Study the drawing (mm; zero at the part's minimum x, y, z) and answer. A direction names the side the tool comes from. Give positions to 0.01 mm unless a question says otherwise; leave off trailing zeros. Write each loop counter-clockwise with the first axis right and the second up, starting at its lowest first coordinate (ties: lowest second). Pieces come first, ordered by that corner, then holes. Notation, with made-up numbers: (-32.5, -30) - (-28.5, -30) arc R9 cw to (-28.5, -18) - close; hole circle Ø10 at (15.5, -38). An arc over 180 degrees is marked (long way). Answer in a Markdown table with one row per item. Add a question column.
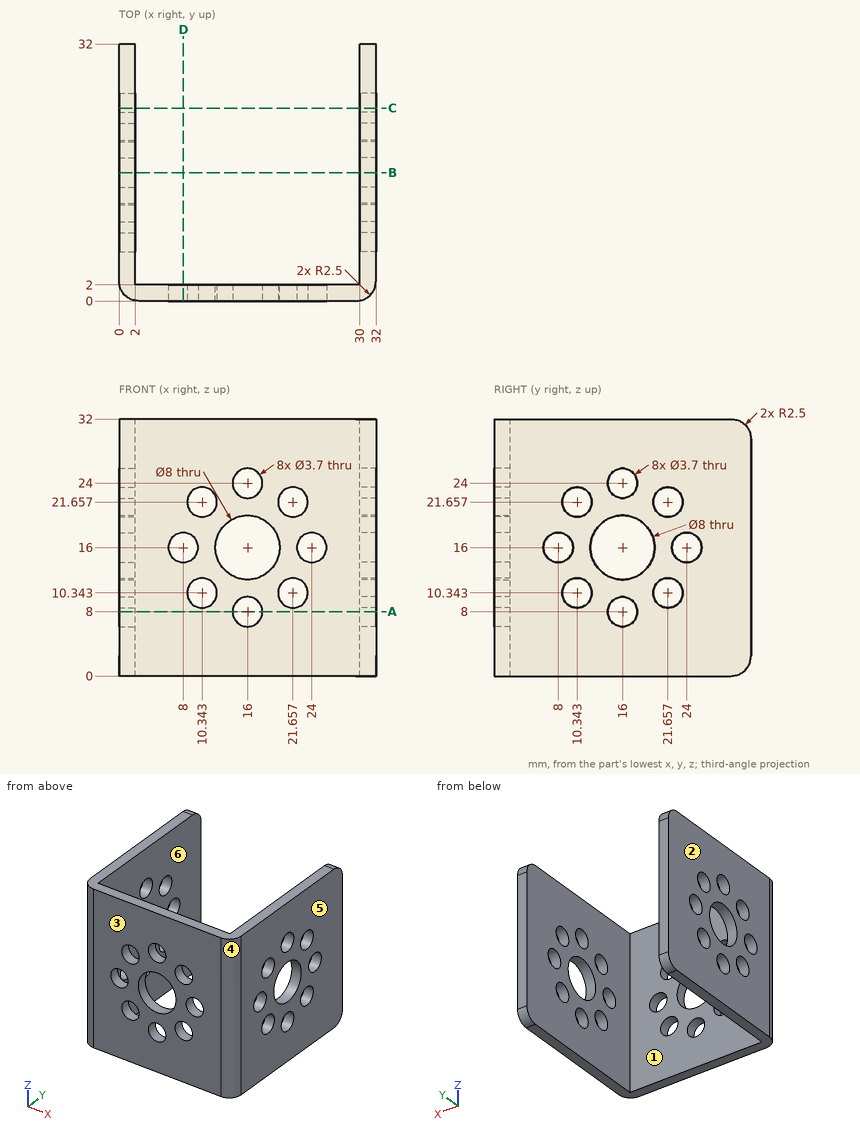
1. Section A-A (z = 8) is taken. Give the vertices of the cut face in (x, y), and give its area (3 significant figures).
2. Section D-D (x = 8) is taken. Give the vertices of the cut face in (y, z), and give its area (3 significant figures).
3. Section B-B (y = 16) is taken. State how many separate pieces and enclosed holes the cut face has, and give its area (3 significant figures).
4. The mould has two halves that part along X. Classify the marked faces 1, 2, 3 and 4: +X half, -X half, draft (parallel to the pull), parting line (faces both ways), or undercut.
5. Given pin 1 Ø3 at (y, z) = (24, 16) entering from -X; pin 2 Ø1 at (x, z) = (17.5, 4) entering from +Y, each flat-ended and moving along its own axis, determine where each tip first touches the part or whether it passes through.
6. Straight lines are drawn through the part: L1, parallel to Z at x = 16, y = 1.05; L2, parallel to X at y = 2.5, z = 2.5; L3, parallel to Y at x = 31, z = 16. For each, find the intervals that lie inside material, in ascending order. Write a range as [from, to].
7. Section C-C (y = 24) is taken. Give the vertices of the cut face in (x, z), and give its area (3 significant figures).
8. A tool of negligible diameter and unlimited length cuts with its end or side. For the marked faces 5 and 6, from which of +Z, -Z, +X, -X, +Y, -Y can it reach the whole face along a straight path? Write none if from no direction.
Geometry check:
| question | item | result |
|---|---|---|
| 1 | outline | (0, 2.5) arc R2.5 ccw to (2.5, 0) - (14.15, 0) - (14.15, 2) - (2, 2) - (2, 14.15) - (0, 14.15) - close; (0, 17.85) - (2, 17.85) - (2, 32) - (0, 32) - close; (17.85, 0) - (29.5, 0) arc R2.5 ccw to (32, 2.5) - (32, 14.15) - (30, 14.15) - (30, 2) - (17.85, 2) - close; (30, 17.85) - (32, 17.85) - (32, 32) - (30, 32) - close |
| 1 | area | 159 mm² |
| 2 | outline | (0, 0) - (2, 0) - (2, 14.15) - (0, 14.15) - close; (0, 17.85) - (2, 17.85) - (2, 32) - (0, 32) - close |
| 2 | area | 56.6 mm² |
| 3 | separate pieces | 8 |
| 3 | enclosed holes | 0 |
| 3 | area | 66.4 mm² |
| 4 | face 1 | undercut |
| 4 | face 2 | -X half |
| 4 | face 3 | draft |
| 4 | face 4 | +X half |
| 5 | pin 1 | through |
| 5 | pin 2 | y = 2 |
| 6 | L1 | [0, 6.15], [9.85, 12], [20, 22.15], [25.85, 32] |
| 6 | L2 | [0, 2], [30, 32] |
| 6 | L3 | [0.5, 6.15], [9.85, 12], [20, 22.15], [25.85, 32] |
| 7 | outline | (0, 0) - (2, 0) - (2, 14.15) - (0, 14.15) - close; (0, 17.85) - (2, 17.85) - (2, 32) - (0, 32) - close; (30, 0) - (32, 0) - (32, 14.15) - (30, 14.15) - close; (30, 17.85) - (32, 17.85) - (32, 32) - (30, 32) - close |
| 7 | area | 113 mm² |
| 8 | face 5 | +Z, -Z, +X, +Y, -Y |
| 8 | face 6 | +Z, -Z, +Y |
